Print and shaded views of the part. All mm, measured from the part's lowest x, y and z. Coordinates: 2 decimals unless noted, no trailing zeros. Order: outer loops, then holes, each group sorted by start corner. A loop starts at its lowest first (then second) coordinate and runs counter-clockwise, first axis right, second up. Notation, with made-up numbers: M 45.5,-20 L 101.5,-20 A24 ccw 101.5,17 Z; hole C 58,-30.5 d2. An arc over 180 degrees is marked long. One line per item, written item: value.
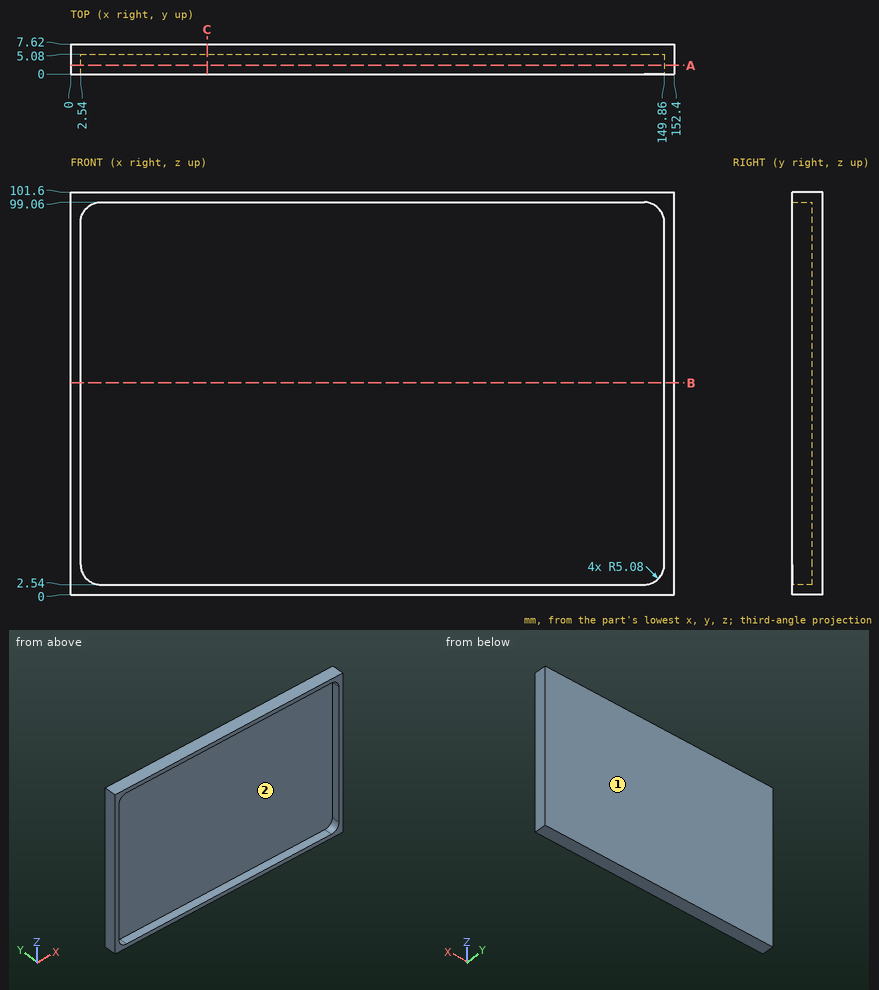
Q1. Drill centre lines: line 1 along X through (y, z) = (2.5, 72); line 2 along Z through (x, y) = (122, 3.75); line 3 along Y through (x, z) = (113, 38). Where is each one in solid material? Low to high.
Recorded:
line 1: x = 0 to 2.54, 149.86 to 152.4
line 2: z = 0 to 2.54, 99.06 to 101.6
line 3: y = 5.08 to 7.62
Q2. Mould opens along Z. For the marked faces 1 and 2 say: released by +Z, released by -Z, zero draft, split by the parting line, or undercut.
Recorded:
face 1: zero draft
face 2: undercut
Q3. Pin check, flat tip, straight feed: pin 1 Ø8 at (x, z) = (96, 51) entering from -Y. Stop position of the tip, or through.
Recorded:
pin 1: stops at y = 5.08
Q4. Slice it at B-B (z = 53.5). List the corners of the cut face in (x, y), plus the area to 3 significant figures.
Recorded:
outline: M 0,0 L 2.54,0 L 2.54,5.08 L 149.86,5.08 L 149.86,0 L 152.4,0 L 152.4,7.62 L 0,7.62 Z
area: 413 mm^2
Q5. Slice it at C-C (x = 34.5). List the corners of the cut face in (y, z), plus the area to 3 significant figures.
Recorded:
outline: M 0,0 L 7.62,0 L 7.62,101.6 L 0,101.6 L 0,99.06 L 5.08,99.06 L 5.08,2.54 L 0,2.54 Z
area: 284 mm^2
Q6. Slice it at A-A (y = 2.25). List the corners of the cut face in (x, z).
Recorded:
outline: M 0,0 L 152.4,0 L 152.4,101.6 L 0,101.6 Z; hole M 2.54,7.62 A5.08 ccw 7.62,2.54 L 144.78,2.54 A5.08 ccw 149.86,7.62 L 149.86,93.98 A5.08 ccw 144.78,99.06 L 7.62,99.06 A5.08 ccw 2.54,93.98 Z
